Autodesk Inventor part; units mm, degrees
ref_plane "YZ Plane" through (0, 0, 0) normal (1, 0, 0) x (0, 1, 0)
ref_plane "XZ Plane" through (0, 0, 0) normal (0, 1, 0) x (-1, 0, 0)
ref_plane "XY Plane" through (0, 0, 0) normal (0, 0, 1) x (1, 0, 0)
sketch "Sketch1" plane through (0, 0, 0) normal (0, 0, 1) x (1, 0, 0)
  circle A0 centre (0, 0) radius 7.5
  dimension "d0" = 15
extrude "Extrusion1" add sketch "Sketch1" along normal blind 10
sketch "Sketch2" plane through (0, 0, 0) normal (0, 0, -1) x (-1, 0, 0)
  circle A0 centre (0, 0) radius 6.5
  circle A1 centre (0, 0) radius 5
  circle A2 centre (0, 0) radius 7.5
  dimension "d3" = 13
  dimension "d4" = 15
  dimension "d5" = 10
extrude "Extrusion2" add sketch "Sketch2" along normal blind 2 contours A0
sketch "Sketch3" plane through (0, 0, 10) normal (0, 0, 1) x (1, 0, 0)
  circle A0 centre (0, 0) radius 7.5
  circle A1 centre (0, 0) radius 2.5
  dimension "d8" = 15
  dimension "d13" = 5
extrude "Extrusion3" add sketch "Sketch3" along normal blind 5 contours A1
properties part number "stredne_koleso"
The listing builds one solid part. Answer for the finished solid, in the listing's coordinates (mm). A direction names the side the tool comes from. Coordinates: 2 decimals unless noted, no trailing zeros. Loops run counter-clockwise (first coordinate to the right, second up) from the corner with the lowest first, then second, coordinate; pieces in that order, holes last.
1) Determine the mould class of faces 1 (the face through (0, 0, 0)), 2 (the face through (-7.493, -0.33, 4.93)), 3 (the face through (1.08, 4.88, -0.99)), 4 (the face through (-6, 3, 0)) for opening direction X: pulls with the +X half, pulls with the -X half, needs draft (parallel to the pull), parting line crosses it, or undercut.
2) Find section C-C on z = -0.5. Write down the section's boundary in (x, y), then the cut area to 3 significant figures.
3) Find the intervals of material crossed by L1, parallel to Y at x = 0, z = -0.45; L2, parallel to Z at x = -1, y = 1.25; L3, parallel to Y at x = -0.25, z = 5.25, in increasing order.
4) Flat-ended cylindrical pins translate along their axes: pin 1 Ø1.5 at (x, z) = (-5.5, 6) entering from +Y; pin 2 Ø3 at (y, z) = (-4.5, 3.5) entering from +X; pin 3 Ø1 at (x, z) = (5, 3) entering from -Y. Find the tip coordinate at first contact, or state that the pin passes through.
5) A tool of negligible diameter and unlimited length cuts with its end or side. For faces 5 (the face through (5.158, 3.955, -0.986)), 6 (the face through (-0.54, 2.44, 12.46)), 7 (the face through (-2, -5, -2)), from which of +Z, -Z, +X, -X, +Y, -Y can it reach the whole face along a straight path? Write none if from no direction.
6) Find section D-D on z = 2.5. Write down the section's boundary in (x, y).
7) Find section A-A on y = 0. Write down the section's boundary in (x, z).
Values:
1. face 1: undercut
1. face 2: parting line crosses it
1. face 3: undercut
1. face 4: needs draft
2. outline: circle Ø13 at (0, 0); hole circle Ø10 at (0, 0)
2. area: 54.2 mm2
3. L1: y = -6.5 to -5, 5 to 6.5
3. L2: z = 0 to 15
3. L3: y = -7.5 to 7.5
4. pin 1: stops at y = 5.8
4. pin 2: stops at x = 6.87
4. pin 3: stops at y = -6
5. face 5: -Z
5. face 6: +Z
5. face 7: -Z, +X, -X, +Y, -Y
6. outline: circle Ø15 at (0, 0)
7. outline: (-7.5, 0) - (-6.5, 0) - (-6.5, -2) - (-5, -2) - (-5, 0) - (5, 0) - (5, -2) - (6.5, -2) - (6.5, 0) - (7.5, 0) - (7.5, 10) - (2.5, 10) - (2.5, 15) - (-2.5, 15) - (-2.5, 10) - (-7.5, 10) - close
